from build123d import *

# Parameters (mm, degrees)
F0_W     = 100
F0_H     = 75
F2_R     = 3
F3_DEPTH = 25


with BuildPart() as f1:
    # F0 (on Front) → F1 (revolve)
    with BuildSketch(Plane.XZ):
        with Locations((-50, -37.5)):
            Rectangle(F0_W, F0_H)
    revolve(axis=Axis((-50, 0, 0), (-1, 0, 0)))

    # F2 (on Right) → F3 (cut)
    with BuildSketch(Plane.YZ):
        with Locations((0, 55)):
            Circle(F2_R)
        with Locations((-47.631397, -27.5)):
            Circle(F2_R)
        with Locations((47.631397, -27.5)):
            Circle(F2_R)
    extrude(amount=-F3_DEPTH, mode=Mode.SUBTRACT)


solid = f1.part
Geometry check sheet. Reference: the model listing, model coordinates, mm. A direction names the side the tool comes from. Coordinates: 2 decimals unless noted, no trailing zeros. Loops run counter-clockwise (first coordinate to the right, second up) from the corner with the lowest first, then second, coordinate; pieces in that order, holes last. Notation, with made-up numbers: (50.5, 24) - (72.5, 24) arc R22 cw to (72.5, 34) - close; hole circle Ø4 at (72.5, 45.5). An arc over 180 degrees is marked (long way). Use one line per item in the form item = value. Start each with the question number.
Item 1: Mould release check, pull along Y, two halves, no side actions. Record for faces 3 (the face through (-49.3, -74.362, 9.764)), 4 (the face through (-12.32, -50.63, -27.37)), 5 (the face through (0, -1, 1)), 6 (the face through (-25, -48, -27)): +Y half, -Y half, draft (parallel to the pull), parting line (faces both ways), or undercut.
Item 2: Thickness scan on probe 1 along Z at (x, y) = (-13, 0); probe 2 along Z at (x, y) = (-49, 53); probe 3 along Y at (x, z) = (-7.5, 26.5). Record the ranges inside material, lowest first.
Item 3: Section check B-B, the plane z = 55. Enter the section's corners in (x, y), and give its area (3 significant figures).
Item 4: Section check C-C, the plane y = -13. Enter the section's corners in (x, z), and give its area (3 significant figures).
Item 5: Section check A-A, the plane x = -23. Enter the section's corners in (y, z), and give its area (3 significant figures).
Item 6: Section check D-D, the plane x = -88. Enter the section's corners in (y, z), and give its area (3 significant figures).
Item 7: Tool access check on faces 1 (the face through (-12.325, 44.634, -27.368)), 2 (the face through (-100, -1, 1)). Record the directions out of +Z, -Z, +X, -X, +Y, -Y that give a thin tool (end or side, any length) a straight path to the whole face; none if there is none.
Item 8: Gauge pin test, flat ends, axial feed: pin 1 (5.5 mm diameter, centred on y = 47.63, z = -27.5, fed in from +X); pin 2 (1.5 mm diameter, centred on x = -57.5, z = 28, fed in from +Y); pin 3 (5 mm diameter, centred on x = -88, z = 38.5, fed in from +Y). Record the tip position at first contact, or that the pin passes through.
Computed:
q1.face_3 = parting line
q1.face_4 = undercut
q1.face_5 = draft
q1.face_6 = undercut
q2.probe_1 = -75 to 52, 58 to 75
q2.probe_2 = -53.07 to 53.07
q2.probe_3 = -70.16 to 70.16
q3.outline = (-100, -50.99) - (0, -50.99) - (0, -3) - (-25, -3) - (-25, 3) - (0, 3) - (0, 50.99) - (-100, 50.99) - close
q3.area = 10,000 mm2
q4.outline = (-100, -73.86) - (0, -73.86) - (0, 73.86) - (-100, 73.86) - close
q4.area = 14,800 mm2
q5.outline = circle Ø150 at (0, 0); hole circle Ø6 at (-47.63, -27.5); hole circle Ø6 at (0, 55); hole circle Ø6 at (47.63, -27.5)
q5.area = 17,600 mm2
q6.outline = circle Ø150 at (0, 0)
q6.area = 17,700 mm2
q7.face_1 = +X
q7.face_2 = +Z, -Z, -X, +Y, -Y
q8.pin_1 = -25
q8.pin_2 = 69.87
q8.pin_3 = 65.8
